Verification items for the finished model (mm, model axes). Face numbers are marked on the shaded views. A direction names the side the tool comes from. Coordinates: 2 decimals unless noted, no trailing zeros. Loops run counter-clockwise (first coordinate to the right, second up) from the corner with the lowest first, then second, coordinate; pieces in that order, holes last. Notation, with made-up numbers: (-25, 70.5) -> (12, 70.5) arc R25 cw to (12, 106.5) -> close; hole circle Ø2 at (61.5, -23). An arc over 180 degrees is marked (long way). Answer as a JSON object with one key per item and string values. Group by question number.
Q1. Gauge pin test, flat ends, axial feed: pin 1 Ø1.5 at (y, z) = (12, 5.5) entering from +X; pin 2 Ø4 at (x, z) = (5.5, 8.5) entering from -Y. Record the tip position at first contact, or that the pin passes through.
Q2. Cross-section at B-B on y = 29. Record the boundary of the cut face in (x, z).
Q3. Set-up check for the marked faces 1 and 2: record each of +Z, -Z, +X, -X, +Y, -Y from which the full face is reachable in a straight line by a thin tool's end or side.
Q4. Cross-section at C-C on z = 8. Record the boundary of the cut face in (x, y).
Q5. Scan lines: L1, parallel to Y at x = 10, z = 5.75; L2, parallel to Z at x = 7.5, y = 7. Record each from-to range of solid material in increasing order.
Q6. Cross-section at A-A on x = 9. Record the boundary of the cut face in (y, z), and give its area (3 significant figures).
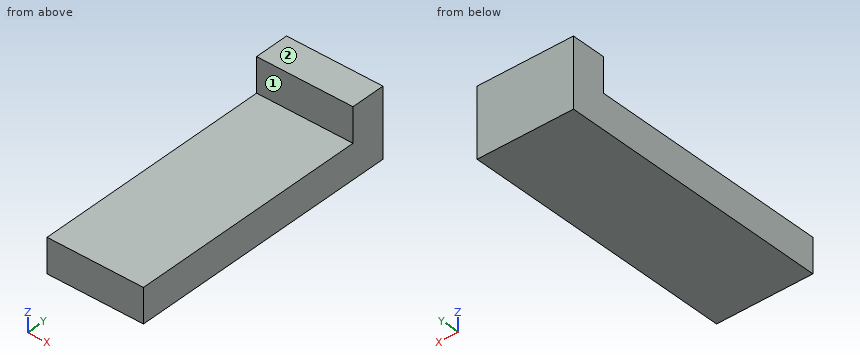
Autodesk Inventor part; units mm, degrees
ref_plane "YZ Plane" through (0, 0, 0) normal (1, 0, 0) x (0, 1, 0)
ref_plane "XZ Plane" through (0, 0, 0) normal (0, 1, 0) x (-1, 0, 0)
ref_plane "XY Plane" through (0, 0, 0) normal (0, 0, 1) x (1, 0, 0)
sketch "Boceto1" plane through (0, 0, 0) normal (0, 0, 1) x (1, 0, 0)
  line L0 (0, 0) -> (14, 0)
  line L1 (14, 0) -> (14, 40)
  line L2 (14, 40) -> (0, 40)
  line L3 (0, 40) -> (0, 0)
  dimension "d0" = 14
  dimension "d1" = 40
extrude "Extrusión1" add sketch "Boceto1" along normal blind 5
sketch "Boceto2" plane through (0, 0, 5) normal (0, 0, 1) x (1, 0, 0)
  line L0 (14, 40) -> (0, 40)
  line L1 (14, 40) -> (0, 40)
  line L2 (0, 40) -> (0, 35)
  line L3 (0, 35) -> (14, 35)
  line L4 (14, 35) -> (14, 40)
  point P0 (0, 0)
  dimension "d4" = 14
  dimension "d5" = 5
extrude "Extrusión2" add sketch "Boceto2" along normal blind 5
properties part number "Pasador"
Computed values:
{
 "1": {"pin 1": "stops at x = 14", "pin 2": "stops at y = 35"},
 "2": {"outline": "(0, 0) -> (14, 0) -> (14, 5) -> (0, 5) -> close"},
 "3": {"face 1": "+Z, +X, -X, -Y", "face 2": "+Z, +X, -X, +Y, -Y"},
 "4": {"outline": "(0, 35) -> (14, 35) -> (14, 40) -> (0, 40) -> close"},
 "5": {"L1": "y = 35 to 40", "L2": "z = 0 to 5"},
 "6": {"outline": "(0, 0) -> (40, 0) -> (40, 10) -> (35, 10) -> (35, 5) -> (0, 5) -> close", "area": "225 mm²"}
}
